from build123d import *

# Parameters (mm, degrees)
SKETCH_1_R               = 19.4
SKETCH_1_R_2             = 17.4
EXTRUDE_1_DEPTH          = 14.5
SKETCH_2_R               = 17.5
SKETCH_2_R_2             = 13.1
EXTRUDE_1_2_DEPTH        = 5.5
SKETCH_3_R               = 13.1
SKETCH_3_R_2             = 12.5
EXTRUDE_2_DEPTH          = 0.5
EXTRUDE_3_DEPTH          = 14.5
CUT_EXTRUDE_1_DEPTH      = 34.143007514
CUT_EXTRUDE_1_DEPTH_BACK = 34.143007514
SKETCH_6_R               = 1
FILLET_1_R               = 1
FILLET_2_R               = 0.5


with BuildPart() as part:
    # 草图1 → Extrude 1 (new body)
    with BuildSketch(Plane(origin=(0, 0, 0), x_dir=(1, 0, 0), z_dir=(0, 1, 0))):
        Circle(SKETCH_1_R)
        Circle(SKETCH_1_R_2, mode=Mode.SUBTRACT)
    extrude(amount=EXTRUDE_1_DEPTH)

    # 草图2 → Extrude 1 2 (add)
    with BuildSketch(Plane(origin=(0, 0, 0), x_dir=(1, 0, 0), z_dir=(0, 1, 0))):
        Circle(SKETCH_2_R)
        with Locations(Location((0, 0, 0), (0, 0, 270))):
            Circle(SKETCH_2_R_2, mode=Mode.SUBTRACT)
    extrude(amount=EXTRUDE_1_2_DEPTH)

    # 草图3 → 凸台-拉伸2 (add)
    with BuildSketch(Plane(origin=(0, 0, 0), x_dir=(1, 0, 0), z_dir=(0, 1, 0))):
        with Locations(Location((0, 0, 0), (0, 0, 270))):
            Circle(SKETCH_3_R)
        with Locations(Location((0, 0, 0), (0, 0, 270))):
            Circle(SKETCH_3_R_2, mode=Mode.SUBTRACT)
    extrude(amount=EXTRUDE_2_DEPTH)

    # 草图4 → 凸台-拉伸3 (add)
    with BuildSketch(Plane(origin=(0, 0, 0), x_dir=(1, 0, 0), z_dir=(0, 1, 0))):
        with BuildLine():
            ThreePointArc((-10, -16.624078922), (-11.553641494, -15.584395023), (-13, -14.4))
            Line((-13, -14.4), (-13, -22.624078922))
            Line((-13, -22.624078922), (-10, -22.624078922))
            Line((-10, -22.624078922), (-10, -16.624078922))
        make_face()
        with BuildLine():
            Line((13, -22.624078922), (13, -14.4))
            ThreePointArc((13, -14.4), (11.553641494, -15.584395023), (10, -16.624078922))
            Line((10, -16.624078922), (10, -22.624078922))
            Line((10, -22.624078922), (13, -22.624078922))
        make_face()
    extrude(amount=EXTRUDE_3_DEPTH)

    # 草图6 → 切除-拉伸1 (cut, two sides: drawn at the far end of the back side and taken through both)
    with BuildSketch(Plane(origin=(0, 0, 0), x_dir=(0, 0, -1), z_dir=(1, 0, 0)).offset(-CUT_EXTRUDE_1_DEPTH_BACK)):
        with Locations((15, 10.5)):
            Circle(SKETCH_6_R)
    extrude(amount=CUT_EXTRUDE_1_DEPTH + CUT_EXTRUDE_1_DEPTH_BACK, mode=Mode.SUBTRACT)

    # 圆角1
    fillet_1_edges = [part.edges().sort_by_distance(p)[0] for p in [
        (-13, 7.25, 22.624078922),
        (-10, 7.25, 22.624078922),
        (13, 7.25, 22.624078922),
        (10, 7.25, 22.624078922),
    ]]
    fillet(fillet_1_edges, radius=FILLET_1_R)

    # 圆角2
    fillet_2_edges = [part.edges().sort_by_distance(p)[0] for p in [
        (0, 5.5, -13.1),
    ]]
    fillet(fillet_2_edges, radius=FILLET_2_R)


solid = part.part
Can you work these out from the model? Positions are in its coordinate system, mm. A direction names the side the tool comes from. Coordinates: 2 decimals unless noted, no trailing zeros. Order: outer loops, then holes, each group sorted by start corner. A loop starts at its lowest first (then second) coordinate and runs counter-clockwise, first axis right, second up. Notation, with made-up numbers: (-30, -20) - (-18, -20) arc R7 cw to (-18, -16) - close; hole circle Ø10 at (28, 77.5). An arc over 180 degrees is marked (long way). Answer as a JSON object with one key per item and string values. Group by question number.
Q1. We'd pull the mould along Z, two halves only. Please class faces 1 (the face through (-10.3, 7.35, 22.34)), 2 (the face through (0.65, 7.15, -19.39)), 3 (the face through (-3.772, 9.937, 16.986)), 4 (the face through (10, 7, 19)): +Z half, -Z half, draft (parallel to the pull), parting line (faces both ways), or undercut.
Q2. Imagine slicing it at C-C (x = 0). Please give me the cut outline in (y, z).
Q3. Imagine slicing it at A-A (z = 20). Please give me the cut outline in (x, y).
Q4. I need wall thicknesses on line 1 (X direction, y = 0.15, z = 0); line 2 (X direction, y = 10, z = 0); line 3 (Z direction, x = 0.5, y = 8). Which ranges of each line are inside material? Lowest first, please. Write a range as from..to.
Q5. Imagine slicing it at D-D (y = 10.5). Please give me the cut outline in (x, z).
Q6. On a 3-axis mill with a long thin cutter (end or side, diameter ignored), from which of +Z, -Z, +X, -X, +Y, -Y can I reach the whole of each face in a straight line? I mean faces 5 (the face through (11.046, 2.718, 7.042)), 6 (the face through (-13, 7, 18)), 7 (the face through (13, 7, 18)). Say none if no direction works.
Q7. Will these pins go through, and if not, where does the flat tip stop? P1, Ø6, axis at x = -13.5, y = 7.5, coming from the -Z side; P2, Ø8, axis at x = -11.5, z = 5, coming from the +Y side; P3, Ø1.5, axis at x = -14, y = 5.5, coming from the +Z side.
Q8. Imagine slicing it at B-B (y = 2.5). Please give me the cut outline in (x, z).
Determined:
{
 "1": {"face 1": "+Z half", "face 2": "parting line", "face 3": "undercut", "face 4": "draft"},
 "2": {"outline": "(0, -19.4) - (14.5, -19.4) - (14.5, -17.4) - (5.5, -17.4) - (5.5, -13.6) arc R0.5 ccw to (5, -13.1) - (0.5, -13.1) - (0.5, -12.5) - (0, -12.5) - close; (0, 12.5) - (0.5, 12.5) - (0.5, 13.1) - (5, 13.1) arc R0.5 ccw to (5.5, 13.6) - (5.5, 17.4) - (14.5, 17.4) - (14.5, 19.4) - (0, 19.4) - close"},
 "3": {"outline": "(-13, 0) - (-10, 0) - (-10, 14.5) - (-13, 14.5) - close; (10, 0) - (13, 0) - (13, 14.5) - (10, 14.5) - close"},
 "4": {"line 1": "x = -19.4..-12.5, 12.5..19.4", "line 2": "x = -19.4..-17.4, 17.4..19.4", "line 3": "z = -19.39..-17.39, 17.39..19.39"},
 "5": {"outline": "(-13.43, -14) - (-10.33, -14) arc R17.4 cw (long way) to (10.33, -14) - (13.43, -14) arc R19.4 ccw to (13, 14.4) - (13, 21.62) arc R1 ccw to (12, 22.62) - (11, 22.62) arc R1 ccw to (10, 21.62) - (10, 16.62) arc R19.4 ccw to (-10, 16.62) - (-10, 21.62) arc R1 ccw to (-11, 22.62) - (-12, 22.62) arc R1 ccw to (-13, 21.62) - (-13, 14.4) arc R19.4 ccw to start; (-10.97, -16) arc R19.4 ccw to (10.97, -16) - (6.84, -16) arc R17.4 cw to (-6.84, -16) - close"},
 "6": {"face 5": "+Y", "face 6": "+Z, -X, +Y, -Y", "face 7": "+Z, +X, +Y, -Y"},
 "7": {"P1": "stops at z = -16.31", "P2": "stops at y = 5.5", "P3": "stops at z = 14.17"},
 "8": {"outline": "(-13, 14.4) arc R19.4 ccw (long way) to (13, 14.4) - (13, 21.62) arc R1 ccw to (12, 22.62) - (11, 22.62) arc R1 ccw to (10, 21.62) - (10, 16.62) arc R19.4 ccw to (-10, 16.62) - (-10, 21.62) arc R1 ccw to (-11, 22.62) - (-12, 22.62) arc R1 ccw to (-13, 21.62) - close; hole circle Ø26.2 at (0, 0)"}
}
